Verification items for the finished model (mm, model axes). Give positions to 0.01 mm unless a question says otherwise; leave off trailing zeros. Write each loop counter-clockwise with the first axis right and the second up, starting at its lowest first coordinate (ties: lowest second). Pieces come first, ordered by that corner, then holes. Notation, with made-up numbers: (9.25, 70.5) - (25.25, 70.5) arc R23 cw to (25.25, 91.5) - close; hole circle Ø11 at (17.25, -26). An arc over 180 degrees is marked (long way). Put each result on its own line as item: value.
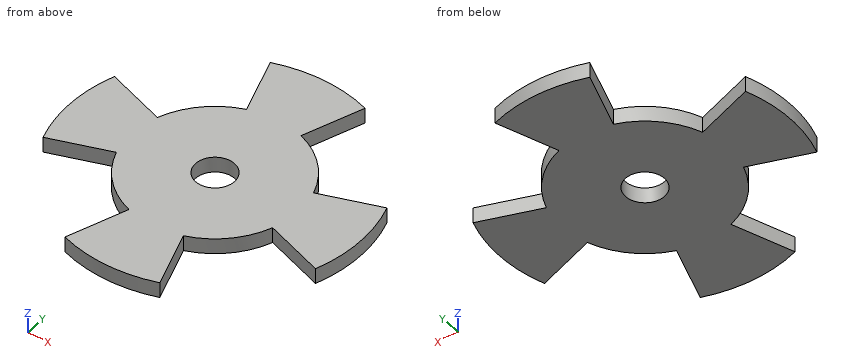
from build123d import *

# Parameters (mm, degrees)
BOSS_EXTRUDE1_DEPTH = 2
SKETCH2_R           = 2.5
CUT_EXTRUDE1_DEPTH  = 27.591822051


with BuildPart() as part:
    # Sketch1 → Boss-Extrude1 (new body)
    with BuildSketch(Plane.XY):
        with BuildLine():
            Line((3.535767004, 10.15188907), (6.167035471, 17.706783262))
            ThreePointArc((6.167035471, 17.706783262), (0, 18.75), (-6.167035471, 17.706783262))
            Line((-6.167035471, 17.706783262), (-3.535767004, 10.15188907))
            ThreePointArc((-3.535767004, 10.15188907), (-7.601397898, 7.601397898), (-10.15188907, 3.535767004))
            Line((-10.15188907, 3.535767004), (-17.706783262, 6.167035471))
            ThreePointArc((-17.706783262, 6.167035471), (-18.75, 0), (-17.706783262, -6.167035471))
            Line((-17.706783262, -6.167035471), (-10.15188907, -3.535767004))
            ThreePointArc((-10.15188907, -3.535767004), (-7.601397898, -7.601397898), (-3.535767004, -10.15188907))
            Line((-3.535767004, -10.15188907), (-6.167035471, -17.706783262))
            ThreePointArc((-6.167035471, -17.706783262), (0, -18.75), (6.167035471, -17.706783262))
            Line((6.167035471, -17.706783262), (3.535767004, -10.15188907))
            ThreePointArc((3.535767004, -10.15188907), (7.601397898, -7.601397898), (10.15188907, -3.535767004))
            Line((10.15188907, -3.535767004), (17.706783262, -6.167035471))
            ThreePointArc((17.706783262, -6.167035471), (18.75, 0), (17.706783262, 6.167035471))
            Line((17.706783262, 6.167035471), (10.15188907, 3.535767004))
            ThreePointArc((10.15188907, 3.535767004), (7.601397898, 7.601397898), (3.535767004, 10.15188907))
        make_face()
    extrude(amount=BOSS_EXTRUDE1_DEPTH)

    # Sketch2 → Cut-Extrude1 (cut, through all)
    with BuildSketch(Plane(origin=(0, 0, 0), x_dir=(-1, 0, 0), z_dir=(0, 0, -1))):
        Circle(SKETCH2_R)
    extrude(amount=-CUT_EXTRUDE1_DEPTH, mode=Mode.SUBTRACT)


solid = part.part
Q1. Section check B-B, the plane z = 0.5. Record the cut outline in (x, y).
Answers follow:
outline: (-17.71, -6.17) - (-10.15, -3.54) arc R10.75 ccw to (-3.54, -10.15) - (-6.17, -17.71) arc R18.75 ccw to (6.17, -17.71) - (3.54, -10.15) arc R10.75 ccw to (10.15, -3.54) - (17.71, -6.17) arc R18.75 ccw to (17.71, 6.17) - (10.15, 3.54) arc R10.75 ccw to (3.54, 10.15) - (6.17, 17.71) arc R18.75 ccw to (-6.17, 17.71) - (-3.54, 10.15) arc R10.75 ccw to (-10.15, 3.54) - (-17.71, 6.17) arc R18.75 ccw to start; hole circle Ø5 at (0, 0)
Q2. Scan lines: line 1 along Y through (x, z) = (0, 0.5); line 2 along Y through (x, z) = (2, 0.8). Record each from-to range of solid material in increasing order.
Answers follow:
line 1: y = -18.75 to -2.5, 2.5 to 18.75
line 2: y = -18.64 to -1.5, 1.5 to 18.64
Q3. Go/stop test with a flat-tipped pin: pin 1 Ø4 at (x, y) = (-10, -10) entering from -Z. Record where the tip stops, or that it passes through.
Answers follow:
pin 1: passes through
Q4. Section check A-A, the plane x = 0. Record the cut outline in (y, z), plus the area to 3 significant figures.
Answers follow:
outline: (-18.75, 0) - (-2.5, 0) - (-2.5, 2) - (-18.75, 2) - close; (2.5, 0) - (18.75, 0) - (18.75, 2) - (2.5, 2) - close
area: 65.0 mm2
Q5. Section check D-D, the plane y = 4.5. Record the cut outline in (x, z).
Answers follow:
outline: (-18.2, 0) - (-12.92, 0) - (-12.92, 2) - (-18.2, 2) - close; (-9.76, 0) - (9.76, 0) - (9.76, 2) - (-9.76, 2) - close; (12.92, 0) - (18.2, 0) - (18.2, 2) - (12.92, 2) - close
